Could you check a few things on this drawing? It's one solid part, dimensions in mm from its lowest x, y, z. A direction names the side the tool comes from. Give positions to 0.01 mm unless a question says otherwise; leave off trailing zeros. Order: outer loops, then holes, each group sorted by start corner. A loop starts at its lowest first (then second) coordinate and runs counter-clockwise, first axis right, second up.
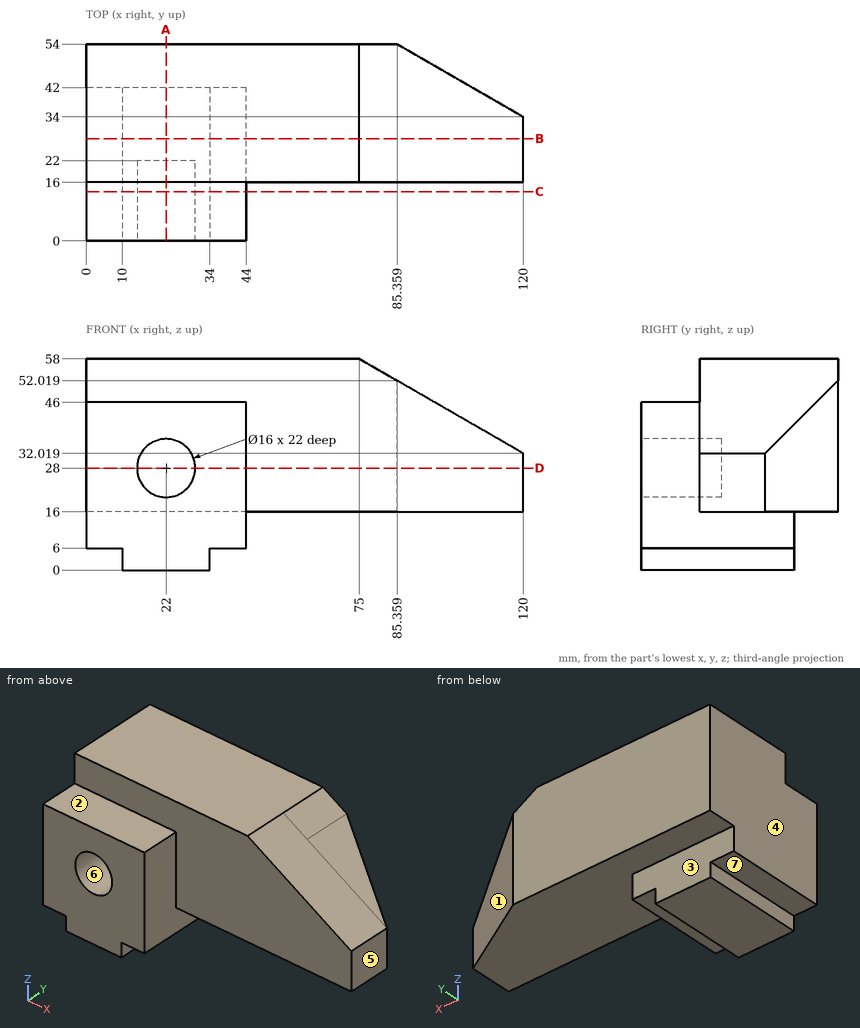
Item 1: Imagine slicing it at D-D on z = 28. List the corners of the cut face in (x, y) for me, then the cut area to 3 significant figures.
Findings:
outline: (0, 0) - (14, 0) - (14, 22) - (30, 22) - (30, 0) - (44, 0) - (44, 16) - (120, 16) - (120, 34) - (85.36, 54) - (0, 54) - close
area: 4,570 mm2
Item 2: Imagine slicing it at B-B on y = 28. List the corners of the cut face in (x, z) for me, then the cut area to 3 significant figures.
Findings:
outline: (0, 6) - (10, 6) - (10, 0) - (34, 0) - (34, 6) - (44, 6) - (44, 16) - (120, 16) - (120, 32.02) - (75, 58) - (0, 58) - close
area: 5,040 mm2
Item 3: For the marked faces 1, 2 and 3, which set-ups out of +Z, -Z, +X, -X, +Y, -Y let a thin tool reach every point of the face, with its end or its side?
Findings:
face 1: +Z, -Z, +X, +Y
face 2: +Z, +X, -X, -Y
face 3: -Z, +X, -X, +Y
Item 4: We'd pull the mould along X, two halves only. Please class the marked faces 4, 5, 6 and 7: +X half, -X half, draft (parallel to the pull), parting line (faces both ways), or undercut.
Findings:
face 4: -X half
face 5: +X half
face 6: undercut
face 7: draft
Item 5: Imagine slicing it at C-C on y = 13.5. List the corners of the cut face in (x, z) for me, then the cut area to 3 significant figures.
Findings:
outline: (0, 6) - (10, 6) - (10, 0) - (34, 0) - (34, 6) - (44, 6) - (44, 46) - (0, 46) - close; hole circle Ø16 at (22, 28)
area: 1,700 mm2
Item 6: Imagine slicing it at A-A on x = 22. List the corners of the cut face in (y, z) for me, then the cut area to 3 significant figures.
Findings:
outline: (0, 0) - (42, 0) - (42, 16) - (54, 16) - (54, 58) - (16, 58) - (16, 46) - (0, 46) - (0, 36) - (22, 36) - (22, 20) - (0, 20) - close
area: 2,400 mm2
Item 7: For pin 1 (18.5 mm diameter, centred on x = 22, z = 28, fed in from -Y); pin 2 (5 mm diameter, centred on y = 22, z = 43.5, fed in from +X) (1 decimal); pin 3 (12 mm diameter, centred on x = 66, z = 39, fed in from -Y); pin 4 (12 mm diameter, centred on y = 48.5, z = 32, fed in from +X), each with a flat end and sliding along its axis, tell me the tip position at first contact or that it passes through.
Findings:
pin 1: stops at y = 0
pin 2: stops at x = 104.4
pin 3: stops at y = 16
pin 4: stops at x = 105.28
Item 8: Please list where these lines run through material, in increasing order: line 1 along Z through (x, y) = (22, 8); line 2 along Y through (x, z) = (69.5, 25); line 3 along Y through (x, z) = (7, 8).
Findings:
line 1: z = 0 to 20, 36 to 46
line 2: y = 16 to 54
line 3: y = 0 to 42
